The model under review builds one solid part; all positions refer to its coordinate system, in mm. Face numbers are marked on the shaded views. A direction names the side the tool comes from. Coordinates: 2 decimals unless noted, no trailing zeros. Order: outer loops, then holes, each group sorted by start corner. A loop starts at its lowest first (then second) coordinate and runs counter-clockwise, first axis right, second up. Notation, with made-up numbers: (-19.5, 8.25) -> (37.5, 8.25) arc R22 ccw to (37.5, 46.25) -> close; hole circle Ø6 at (-20, -20). An arc over 180 degrees is marked (long way). Put each result on its own line as item: value.
from build123d import *

# Parameters (mm, degrees)
F0_R      = 8
F1_DEPTH  = 34
F2_R      = 5.1
F2_R_2    = 1.5
F3_DEPTH  = 50
F4_SIZE   = 1
F6_DEPTH  = 10
F8_DEPTH  = 25
F9_R      = 3.3
F10_DEPTH = 12
F12_R     = 3
F13_DEPTH = 12


with BuildPart() as f1:
    # F0 (on Top) → F1 (new body)
    with BuildSketch(Plane.XY):
        Circle(F0_R)
    extrude(amount=F1_DEPTH)

    # F2 (on Right) → F3 (cut, symmetric)
    with BuildSketch(Plane.YZ):
        with Locations((0, 22)):
            Circle(F2_R)
        with Locations((0, 5)):
            Circle(F2_R_2)
    extrude(amount=F3_DEPTH, both=True, mode=Mode.SUBTRACT)

    # F4
    f4_edges = [f1.edges().sort_by_distance(p)[0] for p in [
        (-8, 0, 34),
    ]]
    chamfer(f4_edges, length=F4_SIZE)

    # F5 (on Top) → F6 (cut)
    with BuildSketch(Plane.XY):
        Polygon((13.330229, -8.80704), (13.330229, 8.80704), (4.25, 8.80704), (4.25, 0), (4.25, -8.80704), align=None)
        Polygon((-4.25, 8.80704), (-13.330229, 8.80704), (-13.330229, -8.80704), (-4.25, -8.80704), (-4.25, 0), align=None)
    extrude(amount=F6_DEPTH, mode=Mode.SUBTRACT)

    # F7 (on face) → F8 (cut)
    with BuildSketch(Plane(origin=(-4.25, 0, 0), x_dir=(0, -1, 0), z_dir=(-1, 0, 0))):
        Polygon((-9.396474, 0), (-4.25, 0), (-9.098946, 4.848946), align=None)
        Polygon((8.720067, 4.470067), (4.25, 0), (10.144616, 0), align=None)
    extrude(amount=-F8_DEPTH, mode=Mode.SUBTRACT)

    # F9 (on Top) → F10 (cut)
    with BuildSketch(Plane.XY):
        Circle(F9_R)
    extrude(amount=-F10_DEPTH, mode=Mode.SUBTRACT)

    # F12 (on face) → F13 (cut)
    with BuildSketch(Plane.XY.offset(34)):
        Circle(F12_R)
    extrude(amount=-F13_DEPTH, mode=Mode.SUBTRACT)


solid = f1.part
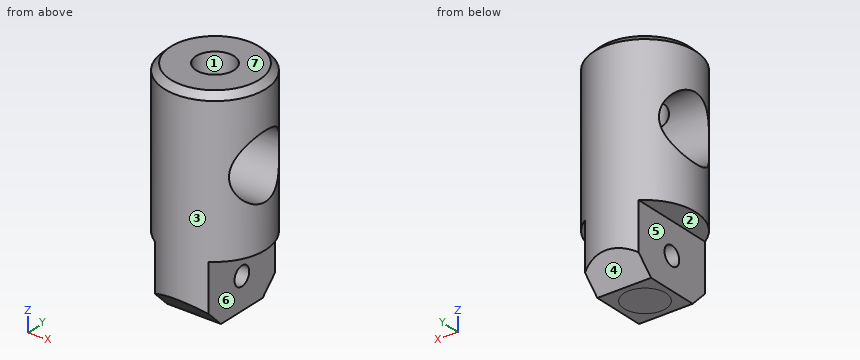
Item 1: For the marked faces 5, 6 and 7, list the 3-axis set-ups (+Z, -Z, +X, -X, +Y, -Y) from which the entire face can be reached by the end or side of a thin tool; tool diameter is ignored.
Answers below:
face 5: -Z, -X, +Y, -Y
face 6: -Z, +X, +Y, -Y
face 7: +Z, +X, -X, +Y, -Y
Item 2: For pin 1 Ø1.1 at (x, y) = (7, 0.5) entering from -Z; pin 2 Ø8 at (y, z) = (2.5, 4) entering from -X; pin 3 Ø1.5 at (y, z) = (-5, 27.5) entering from -X, all flat-tipped, find the tip position at first contact; note any pin that passes through.
Answers below:
pin 1: z = 10
pin 2: x = -4.25
pin 3: x = -6.78
Item 3: Consider section C-C on z = 28. Write out the cut boundary in (x, y), and give its area (3 significant figures).
Answers below:
outline: circle Ø16 at (0, 0); hole circle Ø6 at (0, 0)
area: 173 mm^2
Item 4: Consider section A-A on y = 0. Write out the cut boundary in (x, z).
Answers below:
outline: (-8, 10) -> (-4.25, 10) -> (-4.25, 6.5) -> (4.25, 6.5) -> (4.25, 10) -> (8, 10) -> (8, 16.9) -> (-8, 16.9) -> close; (-8, 27.1) -> (-3, 27.1) -> (-3, 34) -> (-7, 34) -> (-8, 33) -> close; (-4.25, 0) -> (4.25, 0) -> (4.25, 3.5) -> (-4.25, 3.5) -> close; (3, 27.1) -> (8, 27.1) -> (8, 33) -> (7, 34) -> (3, 34) -> close
Item 5: For line 1 (Z direction, x = 4, y = 0); line 2 (Y direction, x = 0, z = 30); line 3 (Z direction, x = -3, y = -0.75), list the stretches that pass through material, from the lowest coordinate up. Write a range as from..to.
Answers below:
line 1: 0..3.5, 6.5..16.9, 27.1..34
line 2: -8..-3, 3..8
line 3: 0..3.7, 6.3..16.96, 27.04..34
Item 6: Consider section B-B on z = 5. Write out the cut boundary in (x, y), and give its area (3 significant figures).
Answers below:
outline: (-4.25, -6.78) arc R8 ccw to (4.25, -6.78) -> (4.25, -1.5) -> (-4.25, -1.5) -> close; (-4.25, 1.5) -> (4.25, 1.5) -> (4.25, 6.78) arc R8 ccw to (-4.25, 6.78) -> close
area: 104 mm^2
Item 7: Mouldability with a two-part tool opening along Y and no side actions: class the marked faces 1, 2, 3 and 4 as +Y half, -Y half, draft (parallel to the pull), parting line (faces both ways), or undercut.
Answers below:
face 1: undercut
face 2: draft
face 3: parting line
face 4: +Y half
Item 8: Consider section D-D on z = 13. Write out the cut boundary in (x, y), and give its area (3 significant figures).
Answers below:
outline: circle Ø16 at (0, 0)
area: 201 mm^2
